Drawing for the job (mm, zero at the part's lowest x, y, z). A direction names the side the tool comes from. Coordinates: 2 decimals unless noted, no trailing zeros. Order: outer loops, then holes, each group sorted by start corner. A loop starts at its lowest first (then second) coordinate and runs counter-clockwise, first axis right, second up. Notation, with made-up numbers: M 33.25,3 L 67.25,3 A20 ccw 67.25,32 Z; hole C 16.25,-20 d6. An arc over 180 degrees is marked long. Write item = value, one per line. Start each with the question number.
Q1. Band-saw the part on B-B on x = 25. Write the cut outline in (y, z), plus the area to 3 significant figures.
Q2. Pin check, flat tips, straight feed: P1, Ø2.5, axis at x = 2, y = 20.5, coming from the -Z side; P2, Ø3, axis at x = 15.5, z = 18, coming from the +Y side; P3, Ø3, axis at x = 40.5, z = 9.5, coming from the +Y side (3 decimals); P4, Ø14, axis at y = 19, z = 27, coming from the +X side. Stop position of each tip, or through.
Q3. 3-axis set-ups, long thin cutter, end or side, ignore diameter. For the marked faces 1 and 2: which of +Z, -Z, +X, -X, +Y, -Y reach the whole face in a straight line?
Q4. Band-saw the part on D-D on z = 31.5. Write the cut outline in (x, y), plus the area to 3 significant figures.
Q5. Band-saw the part on A-A on y = 24. Write the cut outline in (x, z), plus the area to 3 significant figures.
Q6. Band-saw the part on C-C on x = 9.5. Write the cut outline in (y, z).
Q7. Drill centre lines: probe 1 along X at (y, z) = (2.3, 40.5); probe 2 along Y at (x, z) = (8.5, 24). Where is each one in solid material? Low to high.
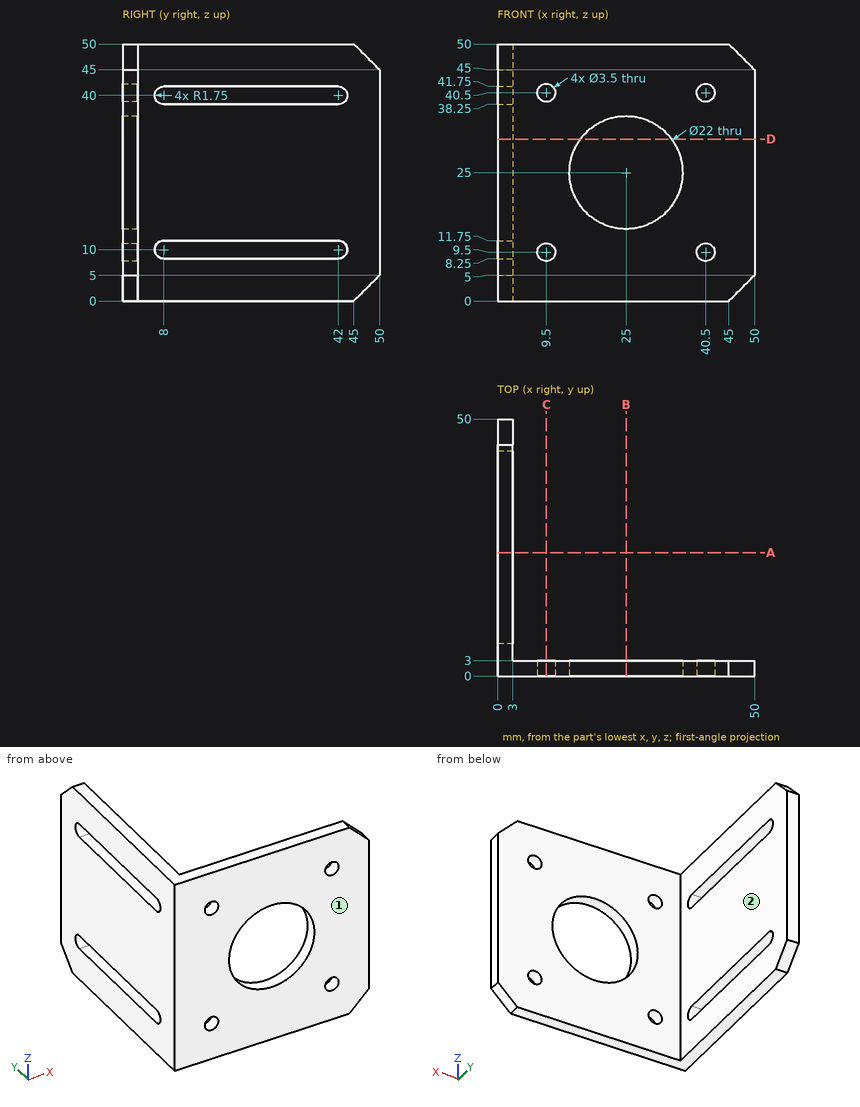
Recorded:
q1.outline = M 0,0 L 3,0 L 3,14 L 0,14 Z; M 0,36 L 3,36 L 3,50 L 0,50 Z
q1.area = 84.0 mm2
q2.P1 = 0
q2.P2 = 3
q2.P3 = through
q2.P4 = 3
q3.face_1 = +Z, -Z, +X, -X, -Y
q3.face_2 = +Z, -Z, +X, +Y
q4.outline = M 0,0 L 16.13,0 L 16.13,3 L 3,3 L 3,50 L 0,50 Z; M 33.87,0 L 50,0 L 50,3 L 33.87,3 Z
q4.area = 238 mm2
q5.outline = M 0,0 L 3,0 L 3,8.25 L 0,8.25 Z; M 0,11.75 L 3,11.75 L 3,38.25 L 0,38.25 Z; M 0,41.75 L 3,41.75 L 3,50 L 0,50 Z
q5.area = 129 mm2
q6.outline = M 0,0 L 3,0 L 3,7.75 L 0,7.75 Z; M 0,11.25 L 3,11.25 L 3,38.75 L 0,38.75 Z; M 0,42.25 L 3,42.25 L 3,50 L 0,50 Z
q7.probe_1 = 0 to 7.75, 11.25 to 38.75, 42.25 to 50
q7.probe_2 = 0 to 3
